Source: CAD feature listing. Evaluate the final solid. Frame: model axes, mm. Give positions to 0.01 mm unless a question says otherwise; leave off trailing zeros. Order: outer loops, then holes, each group sorted by start corner. A loop starts at its lowest first (then second) coordinate and runs counter-clockwise, first axis right, second up.
1) First-contact query: P1, Ø9.5, axis at x = 0, y = 0, coming from the +Z side; P2, Ø1, axis at y = 19.5, z = 4.5, coming from the +X side; P3, Ø5, axis at y = 36.5, z = 6.5, coming from the +X side; P4, Ø3, axis at y = 30, z = 5.5, coming from the +X side. Flat tips, straight axial feed; report the tip coordinate or a pass-through.
2) Section C-C, the plane y = 11.5. Return loops of the section in (x, z), plus the area to 3 significant figures.
3) Section A-A, the plane z = 7.5. Return loops of the section in (x, y) (3 decimals).
4) Section B-B, the plane x = 63. Return loops of the section in (y, z).
5) Material intervals for line 1 (Y direction, x = 0, z = 7.75); line 2 (X direction, y = -1, z = 2.5); line 3 (X direction, y = 2, z = 0.75), sorted ascending.
6) Draft query along X for faces 1 (the face through (-18, 28, 0)), 2 (the face through (74.263, 55.69, 4.93)), 3 (the face through (80.926, 57.838, 4.93)). Return one class per face: released by +X, released by -X, zero draft, split by the parting line, or undercut.
```python
from build123d import *

# Parameters (mm, degrees)
SKETCH2_R      = 10
SKETCH2_R_2    = 3
EXTRUDE1_DEPTH = 10


with BuildPart() as part:
    # Sketch2 → Extrude1 (new body)
    # profile 1 of 5: a face of its own
    with BuildSketch(Plane.XY):
        with BuildLine():
            Line((71.401800626, 64.788528611), (-70, 64.788528611))
            ThreePointArc((-70, 64.788528611), (-62.928932188, 61.859596423), (-60, 54.788528611))
            ThreePointArc((-60, 54.788528611), (-70, 44.788528611), (-80, 54.788528611))
            Line((-80, 54.788528611), (-80, 0))
            ThreePointArc((-80, 0), (-70, 10), (-60, 0))
            ThreePointArc((-60, 0), (-62.928932188, -7.071067812), (-70, -10))
            Line((-70, -10), (0, -10))
            ThreePointArc((0, -10), (-7.071067812, 7.071067812), (10, 0))
            ThreePointArc((10, 0), (8.968727415, -4.422886902), (6.08761429, -7.933533403))
            Line((6.08761429, -7.933533403), (77.489414916, 46.854995208))
            ThreePointArc((77.489414916, 46.854995208), (61.932499331, 51.574133958), (71.401800626, 64.788528611))
        make_face()
    # profile 2 of 5: a face of its own
    with BuildSketch(Plane.XY):
        Circle(SKETCH2_R)
        Circle(SKETCH2_R_2, mode=Mode.SUBTRACT)
    # profile 3 of 5: a face of its own
    with BuildSketch(Plane.XY):
        with Locations((-70, 0)):
            Circle(SKETCH2_R)
    # profile 4 of 5: a face of its own
    with BuildSketch(Plane.XY):
        with Locations((-70, 54.788528611)):
            Circle(SKETCH2_R)
    # profile 5 of 5: a face of its own
    with BuildSketch(Plane.XY):
        with Locations((71.401800626, 54.788528611)):
            Circle(SKETCH2_R)
        with Locations((71.401800626, 54.788528611)):
            Circle(SKETCH2_R_2, mode=Mode.SUBTRACT)
    extrude(amount=EXTRUDE1_DEPTH)


solid = part.part
```
From the geometry:
1. P1: stops at z = 10
1. P2: stops at x = 42.49
1. P3: stops at x = 67.25
1. P4: stops at x = 57.48
2. outline: (-80, 0) - (31.41, 0) - (31.41, 10) - (-80, 10) - close
2. area: 1,110 mm2
3. outline: (-80, 0) arc R10 ccw to (-70, -10) - (0, -10) arc R10 ccw to (6.088, -7.934) - (77.489, 46.855) arc R10 ccw to (71.402, 64.789) - (-70, 64.789) arc R10 ccw to (-80, 54.789) - close; hole circle Ø6 at (0, 0); hole circle Ø6 at (71.402, 54.789)
4. outline: (35.74, 0) - (64.79, 0) - (64.79, 10) - (35.74, 10) - close
5. line 1: y = -10 to -3, 3 to 64.79
5. line 2: x = -79.95 to -2.83, 2.83 to 15.12
5. line 3: x = -80 to -2.24, 2.24 to 19.03
6. face 1: zero draft
6. face 2: undercut
6. face 3: released by +X
